CAD build for the part. Positions are in the model's coordinates, mm. Round coordinates to 2 decimals unless told otherwise and drop trailing zeros. Loops run counter-clockwise (first coordinate to the right, second up) from the corner with the lowest first, then second, coordinate; pieces in that order, holes last.
Autodesk Inventor part; units mm, degrees
ref_plane "YZ Plane" through (0, 0, 0) normal (1, 0, 0) x (0, 1, 0)
ref_plane "XZ Plane" through (0, 0, 0) normal (0, 1, 0) x (-1, 0, 0)
ref_plane "XY Plane" through (0, 0, 0) normal (0, 0, 1) x (1, 0, 0)
sketch "Sketch1" plane through (0, 0, 0) normal (0, 0, 1) x (1, 0, 0)
  line L0 (0, 0) -> (350, 0)
  line L1 (350, 0) -> (350, 260)
  line L2 (350, 260) -> (0, 260)
  line L3 (0, 260) -> (0, 0)
  line L4 (212.725, 66.675) -> (332.725, 66.675)
  line L5 (332.725, 66.675) -> (332.725, 186.675)
  line L6 (332.725, 186.675) -> (212.725, 186.675)
  line L7 (212.725, 186.675) -> (212.725, 66.675)
  circle A0 centre (212.725, 66.675) radius 5
  circle A1 centre (212.725, 186.675) radius 5
  circle A2 centre (332.725, 186.675) radius 5
  circle A3 centre (332.725, 66.675) radius 5
  dimension "d0" = 350
  dimension "d1" = 260
  dimension "d59" = 120
  dimension "d60" = 120
  dimension "d61" = 10
  dimension "d62" = 10
  dimension "d63" = 10
  dimension "d64" = 10
extrude "Extrusion1" add sketch "Sketch1" along normal blind 10 contours L3 L2 L1 L0 | L7 A0 L4 | L4 A0 L7 | A0 L7 A1 L6 A2 L5 A3 L4 | A3 L5 L4 | L4 L5 A3 | A1 L6 L7 | L7 L6 A1 | A2 L6 L5 | L5 L6 A2
sketch "Sketch2" plane through (0, 0, 10) normal (0, 0, 1) x (1, 0, 0)
  line L0 (0, 0) -> (0, 45)
  line L1 (0, 260) -> (0, 0)
  line L2 (0, 260) -> (0, 215)
  line L3 (0, 215) -> (20, 215)
  line L4 (0, 45) -> (20, 45)
  line L5 (20, 45) -> (20, 215)
  dimension "d4" = 45
  dimension "d5" = 45
  dimension "d6" = 20
  dimension "d7" = 20
sketch "Sketch3" plane through (0, 0, 10) normal (0, 0, 1) x (1, 0, 0)
  point P0 (0, 0)
sketch "Sketch4" plane through (0, 0, 10) normal (0, 0, 1) x (1, 0, 0)
  line L0 (0, 0) -> (180, 0)
  line L1 (0, 0) -> (350, 0)
  dimension "d8" = 180
sketch "Sketch5" plane through (0, 0, 10) normal (0, 0, 1) x (1, 0, 0)
  line L0 (19.05, 215.9) -> (179.05, 215.9)
  line L1 (179.05, 215.9) -> (179.05, 55.9)
  line L2 (179.05, 55.9) -> (19.05, 55.9)
  line L3 (19.05, 215.9) -> (38.1, 215.9)
  point P0 (0, 0)
  dimension "d9" = 160
  dimension "d10" = 160
  dimension "d11" = 160
sketch "Sketch6" plane through (0, 0, 10) normal (0, 0, 1) x (1, 0, 0)
  line L0 (20.6375, 215.9) -> (30.6375, 215.9)
  line L1 (30.6375, 215.9) -> (30.6375, 65.9)
  line L2 (30.6375, 65.9) -> (170.6375, 65.9)
  line L3 (170.6375, 65.9) -> (170.6375, 205.9)
  line L4 (170.6375, 205.9) -> (30.6375, 205.9)
  circle A0 centre (30.6375, 205.9) radius 5
  circle A1 centre (170.6375, 205.9) radius 5
  circle A2 centre (30.6375, 65.9) radius 5
  circle A3 centre (170.6375, 65.9) radius 5
  line L5 (212.725, 74.6125) -> (332.725, 74.6125)
  line L6 (332.725, 74.6125) -> (332.725, 194.6125)
  line L7 (332.725, 194.6125) -> (212.725, 194.6125)
  line L8 (212.725, 194.6125) -> (212.725, 74.6125)
  circle A4 centre (212.725, 74.6125) radius 5
  circle A5 centre (212.725, 194.6125) radius 5
  circle A6 centre (332.725, 194.6125) radius 5
  circle A7 centre (332.725, 74.6125) radius 5
  point P0 (0, 0)
  dimension "d12" = 10
  dimension "d13" = 150
  dimension "d14" = 140
  dimension "d15" = 140
  dimension "d16" = 140
  dimension "d17" = 10
  dimension "d18" = 10
  dimension "d19" = 10
  dimension "d20" = 10
  dimension "d65" = 120
  dimension "d66" = 120
  dimension "d67" = 10
  dimension "d68" = 10
  dimension "d69" = 10
  dimension "d70" = 10
extrude "Extrusion2" cut sketch "Sketch6" along normal through all both and the other way through all contours A0 L4 L1 | L1 A0 | L4 A0 L1 | A1 L3 L4 | L4 L3 A1 | A2 L2 L1 | L1 L2 A2 | A3 L2 L3 | L3 L2 A3
sketch "Sketch7" plane through (0, 0, 10) normal (0, 0, 1) x (1, 0, 0)
  circle A0 centre (170.6375, 65.9) radius 5
  line L0 (170.6375, 65.9) -> (190.6375, 65.9)
  line L1 (190.6375, 65.9) -> (190.6375, 225.9)
  line L2 (190.6375, 225.9) -> (190.6375, 204.7875)
  point P0 (0, 0)
  dimension "d23" = 20
  dimension "d24" = 160
sketch "Sketch8" plane through (0, 0, 10) normal (0, 0, 1) x (1, 0, 0)
  line L0 (171.45, 204.7875) -> (190.5, 204.7875)
  line L1 (190.5, 204.7875) -> (190.5, 179.7875)
  point P0 (0, 0)
  dimension "d45" = 25
extrude "Extrusion3" [suppressed]
sketch "Sketch9" plane through (0, 0, 10) normal (0, 0, 1) x (1, 0, 0)
  point P0 (0, 0)
sketch "Sketch10" plane through (0, 0, 0) normal (0, 0, -1) x (-1, 0, 0)
  line L0 (-211.1375, 187.325) -> (-321.1375, 187.325)
  line L1 (-321.1375, 187.325) -> (-321.1375, 77.325)
  line L2 (-321.1375, 77.325) -> (-211.1375, 77.325)
  line L3 (-211.1375, 77.325) -> (-211.1375, 187.325)
  circle A0 centre (-211.1375, 187.325) radius 5
  circle A1 centre (-211.1375, 77.325) radius 5
  circle A2 centre (-321.1375, 77.325) radius 5
  circle A3 centre (-321.1375, 187.325) radius 5
  point P0 (0, 0)
  dimension "d71" = 110
  dimension "d72" = 110
  dimension "d73" = 10
  dimension "d74" = 10
  dimension "d75" = 10
  dimension "d76" = 10
extrude "Extrusion4" cut sketch "Sketch10" against normal through all contours A3 L1 L0 | L0 L1 A3 | A0 L3 L0 | L0 L3 A0 | A2 L2 L1 | L1 L2 A2 | A1 L2 L3 | L3 L2 A1
sketch "Sketch11" plane through (0, 0, 10) normal (0, 0, 1) x (1, 0, 0)
  line L0 (350, 260) -> (450, 260)
  line L1 (450, 260) -> (450, 0)
  line L2 (450, 0) -> (350, 0)
  line L3 (350, 0) -> (350, 260)
  point P0 (0, 0)
  dimension "d79" = 100
extrude "Extrusion5" add sketch "Sketch11" against normal blind 10
sketch "Sketch12" plane through (0, 0, 10) normal (0, 0, 1) x (1, 0, 0)
  point P0 (0, 0)
sketch "Sketch13" plane through (0, 0, 10) normal (0, 0, 1) x (1, 0, 0)
  line L0 (450, 260) -> (450, 0)
  line L1 (450, 0) -> (250.825, 0)
  line L2 (0, 0) -> (450, 0)
sketch "Sketch14" plane through (0, 0, 10) normal (0, 0, 1) x (1, 0, 0)
  line L0 (0, 0) -> (450, 0)
  line L1 (252.4125, 0) -> (252.4125, 20)
  line L2 (450, 0) -> (252.4125, 0)
  line L3 (252.4125, 0) -> (252.4125, 10)
  circle A0 centre (252.4125, 10) radius 5
  line L4 (252.4125, 10) -> (252.4125, 258.7625)
  line L5 (252.4125, 258.7625) -> (252.4125, 248.7625)
  circle A1 centre (252.4125, 248.7625) radius 5
  dimension "d89" = 10
  dimension "d90" = 10
  dimension "d91" = 10
  dimension "d92" = 10
extrude "Extrusion6" [suppressed]
sketch "Sketch15" plane through (0, 0, 10) normal (0, 0, 1) x (1, 0, 0)
  line L0 (0, 0) -> (450, 0)
  line L1 (252.4125, 232.581) -> (252.4125, 242.8875)
extrude "Extrusion7" [suppressed]
sketch "Sketch16" plane through (0, 0, 10) normal (0, 0, 1) x (1, 0, 0)
  line L0 (0, 0) -> (450, 0)
  line L1 (252.4125, 0) -> (-7.5875, 0)
  dimension "d93" = 260
sketch "Sketch17" plane through (0, 0, 10) normal (0, 0, 1) x (1, 0, 0)
  line L0 (250.825, 0) -> (250.825, 10)
  line L1 (250.825, 10) -> (250.825, 250)
  circle A0 centre (250.825, 250) radius 5
  circle A1 centre (250.825, 10) radius 5
  point P0 (0, 0)
  dimension "d94" = 10
  dimension "d95" = 240
  dimension "d96" = 10
  dimension "d97" = 10
extrude "Extrusion8" cut sketch "Sketch17" against normal blind 10
equation "\"d36\" = d29"
equation "\"d98\" = d97"
properties part number "BASE FOR SYSTEM"
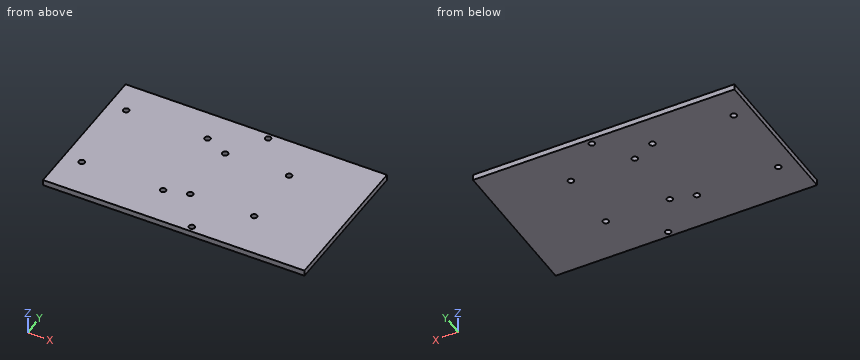
Item 1: Flat gauge pin, fed straight in: P1, Ø8, axis at x = 211.14, y = 77.32, coming from the +Z side. Where does the tip first touch, or does it go through?
Answers follow:
P1: passes through
Item 2: Probe line 1 (X direction, y = 205.9, z = 3); line 2 (X direction, y = 64, z = 6.75). List the from-to ranges inside material, lowest first.
Answers follow:
line 1: x = 0 to 25.64, 35.64 to 165.64, 175.64 to 450
line 2: x = 0 to 26.01, 35.26 to 166.01, 175.26 to 450
Item 3: Cut at B-B, the plane y = 65.9. Give the cut face in (x, z).
Answers follow:
outline: (0, 0) - (25.64, 0) - (25.64, 10) - (0, 10) - close; (35.64, 0) - (165.64, 0) - (165.64, 10) - (35.64, 10) - close; (175.64, 0) - (450, 0) - (450, 10) - (175.64, 10) - close
Item 4: Cut at A-A, the plane y = 10. Give the cut face in (x, z) (3 decimals).
Answers follow:
outline: (0, 0) - (245.825, 0) - (245.825, 10) - (0, 10) - close; (255.825, 0) - (450, 0) - (450, 10) - (255.825, 10) - close
